Read the model definition and answer for the solid it produces. Units are mm, in the model's axes. A direction names the side the tool comes from. Coordinates: 2 decimals unless noted, no trailing zeros. Loops run counter-clockwise (first coordinate to the right, second up) from the corner with the lowest first, then second, coordinate; pieces in that order, holes last.
Q1. Straight lines are drawn through the part: line 1 (Z direction, x = 17, y = 0); line 2 (X direction, y = 0, z = 847); line 3 (Z direction, x = 9.5, y = -19). For each, find the intervals that lie inside material, in ascending order.
Q2. Which of the six approach directions +Z, -Z, +X, -X, +Y, -Y give full straight-line access (tool end or side, diameter ignored) to faces 1 (the face through (8, -8, 938.2)), 2 (the face through (13.5, 14.3, 823.2)), 3 (the face through (-14, 14, 838.2))?
Q3. Section D-D (x = -23) is taken. Give the vertices of the cut face in (y, z).
Q4. Flat-ended cylindrical pins translate along their axes: P1, Ø5, axis at x = -17, z = 862, coming from the -Y side; P2, Ø8, axis at x = 8.5, z = 891.5, coming from the -Y side; P3, Ø1.5, axis at x = -1, z = 916.5, coming from the +Y side; P4, Ø2.5, axis at y = 0, z = 858.2, coming from the +X side. Find the tip coordinate at first contact, or state that the pin passes through.
Q5. Section A-A (y = 0) is taken. Count the separate pieces of the cut face and the enclosed holes in it, then the cut area to 3 significant figures.
Q6. Section C-C (z = 858.2) is taken. Give the vertices of the cut face in (x, y), then the cut area to 3 significant figures.
Q7. The mould has two halves that part along X. Classify faces 4 (the face through (13.827, -25.995, 830.805)), 5 (the face through (-13.827, 25.995, 830.805)), 6 (the face through (8, -8, 815.2)), 7 (the face through (8.767, -16.856, 819.256)): pulls with the +X half, pulls with the -X half, needs draft (parallel to the pull), parting line crosses it, or undercut.
from build123d import *

# Parameters (mm, degrees)
ESQUISSE1_R                  = 2.65
BOSS_EXTRU_1_DEPTH           = 15
ESQUISSE9_R                  = 19
BOSS_EXTRU_4_DEPTH           = 100
BOSS_EXTRU_4_DEPTH_BACK      = 23
ESQUISSE12_R                 = 10
ENL_V_MAT_EXTRU_2_DEPTH      = 124
ESQUISSE13_R                 = 5
ENL_V_MAT_EXTRU_3_DEPTH      = 7
ESQUISSE14_R                 = 1.5
ENL_V_MAT_EXTRU_4_DEPTH      = 32.248101798
ENL_V_MAT_EXTRU_4_DEPTH_BACK = 32.248101798
ESQUISSE15_R                 = 1.5
ENL_V_MAT_EXTRU_5_DEPTH      = 32.248101798
ENL_V_MAT_EXTRU_5_DEPTH_BACK = 32.248101798


with BuildPart() as part:
    # Esquisse1 → Boss.-Extru.1 (new body)
    with BuildSketch(Plane.XY.offset(838.2)):
        with BuildLine():
            ThreePointArc((-9.11861011, 26.177363431), (-13.892343586, 26.012514183), (-17.921893066, 28.577360682))
            ThreePointArc((-17.921893066, 28.577360682), (-29.033821851, 29.033821851), (-28.577360682, 17.921893066))
            ThreePointArc((-28.577360682, 17.921893066), (-26.012514183, 13.892343586), (-26.177363431, 9.11861011))
            ThreePointArc((-26.177363431, 9.11861011), (-19.60106383, -19.60106383), (9.11861011, -26.177363431))
            ThreePointArc((9.11861011, -26.177363431), (13.892343586, -26.012514183), (17.921893066, -28.577360682))
            ThreePointArc((17.921893066, -28.577360682), (29.033821851, -29.033821851), (28.577360682, -17.921893066))
            ThreePointArc((28.577360682, -17.921893066), (26.012514183, -13.892343586), (26.177363431, -9.11861011))
            ThreePointArc((26.177363431, -9.11861011), (19.60106383, 19.60106383), (-9.11861011, 26.177363431))
        make_face()
        with Locations((23.68807717, -23.68807717)):
            Circle(ESQUISSE1_R, mode=Mode.SUBTRACT)
        with Locations((-23.68807717, 23.68807717)):
            Circle(ESQUISSE1_R, mode=Mode.SUBTRACT)
    extrude(amount=-BOSS_EXTRU_1_DEPTH)

    # Esquisse9 → Boss.-Extru.4 (add, two sides)
    with BuildSketch(Plane.XY.offset(838.2)) as boss_extru_4_sk:
        Circle(ESQUISSE9_R)
    extrude(amount=BOSS_EXTRU_4_DEPTH)
    extrude(boss_extru_4_sk.sketch, amount=-BOSS_EXTRU_4_DEPTH_BACK)

    # Esquisse12 → Enlèv. mat.-Extru.2 (cut, through all)
    with BuildSketch(Plane.XY.offset(938.2)):
        Circle(ESQUISSE12_R)
    extrude(amount=-ENL_V_MAT_EXTRU_2_DEPTH, mode=Mode.SUBTRACT)

    # Esquisse13 → Enlèv. mat.-Extru.3 (cut)
    with BuildSketch(Plane.XY.offset(838.2)):
        with Locations((-23.68807717, 23.68807717)):
            Circle(ESQUISSE13_R)
        with Locations((23.68807717, -23.68807717)):
            Circle(ESQUISSE13_R)
    extrude(amount=-ENL_V_MAT_EXTRU_3_DEPTH, mode=Mode.SUBTRACT)

    # Esquisse14 → Enlèv. mat.-Extru.4 (cut, two sides)
    with BuildSketch(Plane(origin=(0, 0, 0), x_dir=(1, 0, 0), z_dir=(0, 1, 0))) as enl_v_mat_extru_4_sk:
        with Locations((0, -858.2)):
            Circle(ESQUISSE14_R)
        with Locations((0, -908.2)):
            Circle(ESQUISSE14_R)
    extrude(amount=ENL_V_MAT_EXTRU_4_DEPTH, mode=Mode.SUBTRACT)
    extrude(enl_v_mat_extru_4_sk.sketch, amount=-ENL_V_MAT_EXTRU_4_DEPTH_BACK, mode=Mode.SUBTRACT)

    # Esquisse15 → Enlèv. mat.-Extru.5 (cut, two sides)
    with BuildSketch(Plane(origin=(0, 0, 0), x_dir=(0, 0, -1), z_dir=(1, 0, 0))) as enl_v_mat_extru_5_sk:
        with Locations((-858.2, 0)):
            Circle(ESQUISSE15_R)
        with Locations((-908.2, 0)):
            Circle(ESQUISSE15_R)
    extrude(amount=ENL_V_MAT_EXTRU_5_DEPTH, mode=Mode.SUBTRACT)
    extrude(enl_v_mat_extru_5_sk.sketch, amount=-ENL_V_MAT_EXTRU_5_DEPTH_BACK, mode=Mode.SUBTRACT)


solid = part.part
Numbers:
1. line 1: z = 815.2 to 856.7, 859.7 to 906.7, 909.7 to 938.2
1. line 2: x = -19 to -10, 10 to 19
1. line 3: z = 823.2 to 838.2
2. face 1: +Z, +X, -X, +Y, -Y
2. face 2: -Z
2. face 3: +Z
3. outline: (-15.47, 823.2) - (21.13, 823.2) - (21.13, 831.2) - (18.74, 831.2) - (18.74, 838.2) - (-15.47, 838.2) - close; (26.25, 823.2) - (31.22, 823.2) - (31.22, 838.2) - (28.64, 838.2) - (28.64, 831.2) - (26.25, 831.2) - close
4. P1: stops at y = -12.28
4. P2: stops at y = -18.46
4. P3: stops at y = 19
4. P4: passes through
5. separate pieces: 6
5. enclosed holes: 0
5. area: 2,370 mm2
6. outline: (-18.94, -1.5) arc R19 ccw to (-1.5, -18.94) - (-1.5, -9.89) arc R10 cw to (-9.89, -1.5) - close; (-18.94, 1.5) - (-9.89, 1.5) arc R10 cw to (-1.5, 9.89) - (-1.5, 18.94) arc R19 ccw to start; (1.5, -18.94) arc R19 ccw to (18.94, -1.5) - (9.89, -1.5) arc R10 cw to (1.5, -9.89) - close; (1.5, 9.89) arc R10 cw to (9.89, 1.5) - (18.94, 1.5) arc R19 ccw to (1.5, 18.94) - close
6. area: 712 mm2
7. face 4: undercut
7. face 5: undercut
7. face 6: needs draft
7. face 7: parting line crosses it
